from build123d import *

# Parameters (mm, degrees)
SKETCH1_W                  = 44.45
SKETCH1_H                  = 101.6
BOSS_EXTRUDE2_DEPTH        = 6.35
FILLET1_R                  = 12.7
F_7_0_201_DIAMETER_HOLE2_D = 5.1054
CUT_EXTRUDE1_DEPTH         = 112.079633597
M4_CLEARANCE_HOLE1_D       = 4.5


with BuildPart() as part:
    # Sketch1 → Boss-Extrude2 (new body)
    with BuildSketch(Plane.XY):
        with Locations((-22.225, 50.8)):
            Rectangle(SKETCH1_W, SKETCH1_H)
    extrude(amount=BOSS_EXTRUDE2_DEPTH)

    # Fillet1
    fillet1_edges = [part.edges().sort_by_distance(p)[0] for p in [
        (0, 0, 3.175),
        (-44.45, 0, 3.175),
    ]]
    fillet(fillet1_edges, radius=FILLET1_R)

    # #7 (0.201) Diameter Hole2 (through all)
    with Locations(Plane(origin=(0, 0, 0), x_dir=(-1, 0, 0), z_dir=(0, 0, -1))):
        with Locations((22.225, 88.9), (22.225, 69.85)):
            Hole(F_7_0_201_DIAMETER_HOLE2_D / 2)

    # Sketch14 → Cut-Extrude1 (cut, through all)
    with BuildSketch(Plane.XY.offset(6.35)):
        Polygon((-14.892651581, 25.4), (-18.558825791, 31.75), (-25.891174209, 31.75), (-29.557348419, 25.4), (-25.891174209, 19.05), (-18.558825791, 19.05), align=None)
    extrude(amount=-CUT_EXTRUDE1_DEPTH, mode=Mode.SUBTRACT)

    # M4 Clearance Hole1 (through all)
    with Locations(Plane(origin=(0, 0, 0), x_dir=(-1, 0, 0), z_dir=(0, 0, -1))):
        with Locations((11.29679677, 28.32820323), (25.15320323, 36.32820323), (33.15320323, 22.47179677), (19.29679677, 14.47179677)):
            Hole(M4_CLEARANCE_HOLE1_D / 2)


solid = part.part
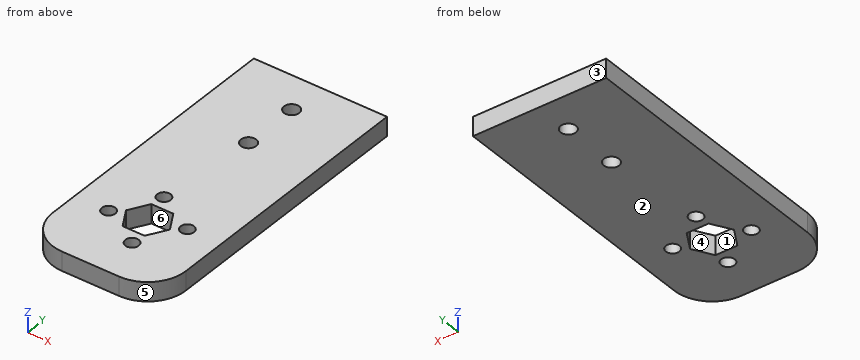
Build history of the part. All positions in model axes, mm. Face numbers are marked on the shaded views. A direction names the side the tool comes from. Round coordinates to 2 decimals unless told otherwise and drop trailing zeros. Write each loop counter-clockwise with the first axis right and the second up, starting at its lowest first coordinate (ties: lowest second). Pieces come first, ordered by that corner, then holes. Notation, with made-up numbers: (27, 19.25) -> (78, 19.25) arc R24 ccw to (78, 30.25) -> close; hole circle Ø6 at (-8, 64.5). An arc over 180 degrees is marked (long way). Write item = value, one per line.
(1) Flat gauge pin, fed straight in: pin 1 (5 mm diameter, centred on x = -19.3, y = 14.47, fed in from +Z). Where does the tip first touch, or does it go through?
Answer:
pin_1 = 6.35
(2) Band-saw the part on A-A (y = 88.9). Give the cut face in (x, z).
Answer:
outline = (-44.45, 0) -> (-24.78, 0) -> (-24.78, 6.35) -> (-44.45, 6.35) -> close; (-19.67, 0) -> (0, 0) -> (0, 6.35) -> (-19.67, 6.35) -> close
(3) Probe L1, parallel to Y at x = -22, z = 4.5; L2, parallel to Y at x = -26, z = 5.5; L3, parallel to X at y = 14, z = 2.75. List the from-to ranges inside material, lowest first.
Answer:
L1 = 0 to 19.05, 31.75 to 67.31, 72.39 to 86.36, 91.44 to 101.6
L2 = 0 to 19.24, 31.56 to 34.24, 38.41 to 101.6
L3 = -44.45 to -21.5, -17.1 to 0
(4) Band-saw the part on D-D (x = -5.5). Give the cut face in (y, z), then the cut area to 3 significant figures.
Answer:
outline = (2.24, 0) -> (101.6, 0) -> (101.6, 6.35) -> (2.24, 6.35) -> close
area = 631 mm2
(5) Two-plate mould, pull along Y, no slides. Class the marked faces 3, 4, 5 and 6: pulls with the +Y half, pulls with the -Y half, needs draft (parallel to the pull), parting line crosses it, or undercut.
Answer:
face_3 = pulls with the +Y half
face_4 = undercut
face_5 = pulls with the -Y half
face_6 = undercut
(6) Band-saw the part on B-B (x = -10). Give the cut face in (y, z).
Answer:
outline = (0.29, 0) -> (26.49, 0) -> (26.49, 6.35) -> (0.29, 6.35) -> close; (30.17, 0) -> (101.6, 0) -> (101.6, 6.35) -> (30.17, 6.35) -> close
(7) Tool access for the marked faces 1 and 2: list every direction of +Z, -Z, +X, -X, +Y, -Y with a clear straight run to the whole face (end or side of a thin tool).
Answer:
face_1 = +Z, -Z
face_2 = -Z, +X, -X, +Y, -Y
(8) Band-saw the part on C-C (z = 1.5). Give the cut face in (x, y) (3 decimals).
Answer:
outline = (-44.45, 12.7) arc R12.7 ccw to (-31.75, 0) -> (-12.7, 0) arc R12.7 ccw to (0, 12.7) -> (0, 101.6) -> (-44.45, 101.6) -> close; hole circle Ø4.5 at (-33.153, 22.472); hole (-29.557, 25.4) -> (-25.891, 19.05) -> (-18.559, 19.05) -> (-14.893, 25.4) -> (-18.559, 31.75) -> (-25.891, 31.75) -> close; hole circle Ø4.5 at (-25.153, 36.328); hole circle Ø5.105 at (-22.225, 69.85); hole circle Ø5.105 at (-22.225, 88.9); hole circle Ø4.5 at (-19.297, 14.472); hole circle Ø4.5 at (-11.297, 28.328)
